Read the model definition and answer for the solid it produces. Units are mm, in the model's axes. A direction names the side the tool comes from. Coordinates: 2 decimals unless noted, no trailing zeros. Order: outer loops, then holes, each group sorted by start corner. A loop starts at its lowest first (then second) coordinate and runs counter-clockwise, first axis right, second up. Notation, with made-up numbers: M 52.5,3.5 L 111.5,3.5 A22 cw 111.5,27.5 Z; hole C 79,11.25 d2. An arc over 180 degrees is marked long. Use a Markdown table: item, result. Add a question column.
1) Find section B-B on y = 74. Write down the section's boundary in (x, z), plus the area to 3 significant figures.
2) The mould has two halves that part along X. Classify faces 1 (the face through (-15.795, 24.559, 7.944)), 2 (the face through (-1, 59, 12)), 3 (the face through (12.54, 79.17, 1.86)): released by +X, released by -X, zero draft, split by the parting line, or undercut.
3) Find the intervals of material crossed by probe 1 along Y at (x, z) = (-6, 5); probe 2 along Y at (x, z) = (1, -6.25); probe 3 along Y at (x, z) = (10, 1.1), in increasing order. Write a range as [from, to].
4) Each of these flat-tipped pins is pushed along its axis until it touches: pin 1 Ø4 at (x, y) = (0, -10) entering from +Z; pin 2 Ø10 at (x, y) = (3, 37) entering from +Z; pin 3 Ø4 at (x, z) = (-6, -5) entering from -Y; pin 4 Ø5 at (y, z) = (62.5, 1.5) entering from -X. Where does it stop, or does it pass through?
5) For faces 4 (the face through (-4.495, 26.623, 7.944)), 5 (the face through (11.23, 92.62, 1.86)), 6 (the face through (12.8, 65, 2)), determine the directions among +Z, -Z, +X, -X, +Y, -Y from which every point of the face is accessible in a straight line to the end or side of a thin tool.
6) Find section C-C on y = 0. Write down the section's boundary in (x, z).
7) Find section D-D on y = 15. Write down the section's boundary in (x, z), plus the area to 3 significant figures.
8) Find section A-A on z = 8.5. Count the separate pieces of the cut face and the enclosed holes in it, plus the area to 3 significant figures.
from build123d import *
from build123d.topology import SkipClean

# Parameters (mm, degrees)
SKETCH_1_R           = 15
SKETCH_1_R_2         = 6.5
SKETCH_1_R_3         = 1.6
EXTRUDE_1_DEPTH      = 4
EXTRUDE_START        = -4
EXTRUDE_3_DEPTH      = 4
EXTRUDE_4_DEPTH      = 8
EXTRUDE_4_DEPTH_BACK = 12
CUT_EXTRUDE_1_DEPTH  = 46


with BuildPart() as part:
    # 草图1 → 凸台-拉伸1 (new body)
    with BuildSketch(Plane.XY):
        Circle(SKETCH_1_R)
        Circle(SKETCH_1_R_2, mode=Mode.SUBTRACT)
        with Locations((0, 10)):
            Circle(SKETCH_1_R_3, mode=Mode.SUBTRACT)
        with Locations((10, 0)):
            Circle(SKETCH_1_R_3, mode=Mode.SUBTRACT)
        with Locations((0, -10)):
            Circle(SKETCH_1_R_3, mode=Mode.SUBTRACT)
        with Locations((-10, 0)):
            Circle(SKETCH_1_R_3, mode=Mode.SUBTRACT)
    extrude(amount=EXTRUDE_1_DEPTH)

    # 草图2 → 凸台-拉伸3 (add)
    with BuildSketch(Plane.XY.offset(4).offset(EXTRUDE_START)):
        with BuildLine():
            Line((16.8, 85), (16.8, 54.159799849))
            ThreePointArc((16.8, 54.159799849), (15.83854762, 48.033324147), (13.046629547, 42.49587991))
            ThreePointArc((13.046629547, 42.49587991), (7.420814059, 25.504374344), (12.472191289, 8.333333333))
            ThreePointArc((12.472191289, 8.333333333), (-5.937882388, 13.774670695), (-14.621995932, -3.346226976))
            ThreePointArc((-14.621995932, -3.346226976), (-15.737901413, 44.738127218), (2.117573463, 89.398315084))
            ThreePointArc((2.117573463, 89.398315084), (11.095712057, 92.663530919), (16.8, 85))
        make_face()
    extrude(amount=EXTRUDE_3_DEPTH)

    # 草图3 → 凸台-拉伸4 (add, two sides: drawn at the far end of the back side and taken through both)
    with SkipClean():  # the faces are left unmerged after this step: merging them gives an invalid solid
        with BuildSketch(Plane.XY.offset(4).offset(-EXTRUDE_4_DEPTH_BACK)):
            with BuildLine():
                Line((16.8, 54.159799849), (16.8, 85))
                ThreePointArc((16.8, 85), (11.095712057, 92.663530919), (2.117573463, 89.398315084))
                ThreePointArc((2.117573463, 89.398315084), (-11.916705707, 60.059804871), (-17.55757213, 28.030290369))
                ThreePointArc((-17.55757213, 28.030290369), (-15.746673, 24.526996644), (-11.810776072, 24.27973576))
                ThreePointArc((-11.810776072, 24.27973576), (-4.386649325, 26.64127076), (3.402697603, 26.784727906))
                ThreePointArc((3.402697603, 26.784727906), (6.286614818, 27.53779516), (7.849127177, 30.076031539))
                ThreePointArc((7.849127177, 30.076031539), (9.742150736, 36.581291134), (13.046629547, 42.49587991))
                ThreePointArc((13.046629547, 42.49587991), (15.83854762, 48.033324147), (16.8, 54.159799849))
            make_face()
        extrude(amount=EXTRUDE_4_DEPTH + EXTRUDE_4_DEPTH_BACK)
    add(part.part.scale(1), mode=Mode.REPLACE)  # the faces are merged on a copy

    # 草图5 → 切除-拉伸1 (cut)
    with BuildSketch(Plane(origin=(0, 0, -8), x_dir=(-1, 0, 0), z_dir=(0, 0, -1))):
        with BuildLine():
            Line((-12.8, 69.762395693), (-12.8, 60.082793322))
            ThreePointArc((-12.8, 60.082793322), (-11.947152873, 58.444489233), (-10.115959713, 58.20340808))
            Line((-10.115959713, 58.20340808), (0.167044148, 61.946115404))
            ThreePointArc((0.167044148, 61.946115404), (1.475393257, 63.65118916), (0.483003861, 65.557551453))
            Line((0.483003861, 65.557551453), (-9.8, 71.494446501))
            ThreePointArc((-9.8, 71.494446501), (-11.8, 71.494446501), (-12.8, 69.762395693))
        make_face()
        with BuildLine():
            Line((-11.8, 78.422649731), (-1.206357847, 72.306407582))
            ThreePointArc((-1.206357847, 72.306407582), (1.162211364, 72.580028303), (1.585705551, 74.926438557))
            ThreePointArc((1.585705551, 74.926438557), (-1.749223409, 81.170317372), (-5.458786731, 87.199157542))
            ThreePointArc((-5.458786731, 87.199157542), (-9.947856029, 88.83176546), (-12.8, 85))
            Line((-12.8, 85), (-12.8, 80.154700538))
            ThreePointArc((-12.8, 80.154700538), (-12.532050808, 79.154700538), (-11.8, 78.422649731))
        make_face()
        with BuildLine():
            Line((5.01005666, 58.38793894), (-5.776995128, 54.461773174))
            ThreePointArc((-5.776995128, 54.461773174), (-7.091051284, 52.669626708), (-5.938191364, 50.769772359))
            Line((-5.938191364, 50.769772359), (7.453099332, 44.525310955))
            ThreePointArc((7.453099332, 44.525310955), (9.539258698, 44.76945259), (10.256783773, 46.743490028))
            ThreePointArc((10.256783773, 46.743490028), (9.051891671, 51.949605837), (7.60645214, 57.094128298))
            ThreePointArc((7.60645214, 57.094128298), (6.586103601, 58.298616303), (5.01005666, 58.38793894))
        make_face()
        with BuildLine():
            Line((-2.123332063, 32.377143259), (7.681973135, 35.004466868))
            ThreePointArc((7.681973135, 35.004466868), (9.156724441, 36.762007035), (8.009571568, 38.748934095))
            Line((8.009571568, 38.748934095), (-5.543860738, 45.069003373))
            ThreePointArc((-5.543860738, 45.069003373), (-7.869208523, 44.601479118), (-8.112845962, 42.242144033))
            ThreePointArc((-8.112845962, 42.242144033), (-6.056960525, 38.136767143), (-4.572948137, 33.791828527))
            ThreePointArc((-4.572948137, 33.791828527), (-3.641181599, 32.577066199), (-2.123332063, 32.377143259))
        make_face()
    extrude(amount=-CUT_EXTRUDE_1_DEPTH, mode=Mode.SUBTRACT)


solid = part.part
Check result:
| question | item | result |
|---|---|---|
| 1 | outline | M -6.47,-8 L -1.79,-8 L -1.79,12 L -6.47,12 Z; M 4.14,-8 L 16.8,-8 L 16.8,12 L 4.14,12 Z |
| 1 | area | 347 mm2 |
| 2 | face 1 | split by the parting line |
| 2 | face 2 | zero draft |
| 2 | face 3 | undercut |
| 3 | probe 1 | y = [26.32, 34.55], [39.69, 45.2], [58.49, 74.99] |
| 3 | probe 2 | y = [26.98, 32.68], [42.95, 48.47], [56.2, 61.52], [66.41, 72.2], [79.84, 87.67] |
| 3 | probe 3 | y = [-11.18, -1.6], [1.6, 12.82], [37.18, 58.25], [71.6, 77.38], [88.82, 92.91] |
| 4 | pin 1 | stops at z = 4 |
| 4 | pin 2 | stops at z = 12 |
| 4 | pin 3 | stops at y = 25.79 |
| 4 | pin 4 | stops at x = -11.94 |
| 5 | face 4 | +Z, -Y |
| 5 | face 5 | +Z, -Z, +Y |
| 5 | face 6 | +Z, -Z |
| 6 | outline | M -15.34,0 L -11.6,0 L -11.6,4 L -15.34,4 Z; M -8.4,0 L -6.5,0 L -6.5,4 L -8.4,4 Z; M 6.5,0 L 8.4,0 L 8.4,4 L 6.5,4 Z; M 11.6,0 L 15,0 L 15,4 L 11.6,4 Z |
| 7 | outline | M -17.35,0 L 9.13,0 L 9.13,4 L -17.35,4 Z |
| 7 | area | 106 mm2 |
| 8 | separate pieces | 1 |
| 8 | enclosed holes | 4 |
| 8 | area | 1,110 mm2 |
